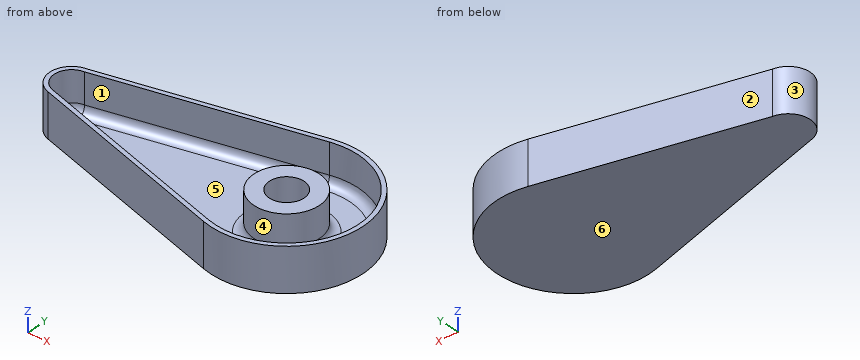
from build123d import *

# Parameters (mm, degrees)
F1_DEPTH = 25.4
F2_T     = -2.54
F3_R     = 19.05
F3_R_2   = 10.16
F4_DEPTH = 22.86
F5_R     = 5.08


with BuildPart() as f1:
    # F0 (on Top) → F1 (new body)
    with BuildSketch(Plane.XY):
        with BuildLine():
            Line((-130.175, -12.2967221242), (-11.1125, -43.0385274347))
            ThreePointArc((-11.1125, -43.0385274347), (44.4499974135, 0.0151638522), (-11.1418620852, 43.0309354915))
            Line((-11.1418620852, 43.0309354915), (-128.75155606, 12.578634718))
            ThreePointArc((-128.75155606, 12.578634718), (-139.6792579893, 0.7255458912), (-130.175, -12.2967221242))
        make_face()
    extrude(amount=F1_DEPTH)

    # F2
    f2_openings = [f1.faces().sort_by_distance(p)[0] for p in [
        (-33.44475, -0.010622, 25.4),
    ]]
    offset(amount=F2_T, openings=f2_openings, kind=Kind.INTERSECTION)

    # F3 (on face) → F4 (join, through all)
    with BuildSketch(Plane.XY.offset(2.54)):
        Circle(F3_R)
        Circle(F3_R_2, mode=Mode.SUBTRACT)
    extrude(amount=F4_DEPTH)

    # F5
    f5_edges = [f1.edges().sort_by_distance(p)[0] for p in [
        (-19.05, 0, 2.54),
        (-69.384764, 25.326524, 2.54),
        (41.909998, 0.014297, 2.54),
        (-137.139228, 0.649358, 2.54),
        (-70.00875, -25.20828, 2.54),
    ]]
    fillet(f5_edges, radius=F5_R)


solid = f1.part
Model file for the job. Use its own axes, mm. Face numbers are marked on the shaded views. A direction names the side the tool comes from. Give positions to 0.01 mm unless a question says otherwise; leave off trailing zeros.
Item 1: Slice it at A-A (z = 18.25). Give the number of separate pieces and of enclosed holes in the cut face, plus the area to 3 significant figures.
Check values:
separate pieces: 2
enclosed holes: 2
area: 1,920 mm2
Item 2: Drill centre lines: line 1 along Y through (x, z) = (0, 20.5); line 2 along X through (y, z) = (-0.5, 7.75); line 3 along Y through (x, z) = (0.5, 17.5). Where is each one in solid material? Low to high.
Check values:
line 1: y = -44.45 to -41.91, -19.05 to -10.16, 10.16 to 19.05, 41.91 to 44.45
line 2: x = -139.69 to -137.15, -19.04 to -10.15, 10.15 to 19.04, 41.91 to 44.45
line 3: y = -44.45 to -41.91, -19.04 to -10.15, 10.15 to 19.04, 41.91 to 44.45
Item 3: Mould opens along Y. For the marked faces 3, 4, 5 and 6 say: +Y half, -Y half, draft (parallel to the pull), parting line (faces both ways), or undercut.
Check values:
face 3: parting line
face 4: undercut
face 5: undercut
face 6: draft
Item 4: Which spindle directions (+Z, -Z, +X, -X, +Y, -Y) get a long thin tool onto all of the face, cutting with end or side? Do the marked faces 1 and 2. Say none if no direction does.
Check values:
face 1: +Z
face 2: +Z, -Z, -X, +Y
Item 5: Drop flat-ended pins along their axis: P1, Ø22, axis at x = -70.5, y = -8, coming from the +Z side; P2, Ø5, axis at x = -7, z = 8, coming from the +Y side; P3, Ø12, axis at x = -22, z = 5.5, coming from the +Y side. Give the stop position or say it passes through.
Check values:
P1: stops at z = 2.54
P2: stops at y = 44.22
P3: stops at y = 41.77
